Autodesk Inventor part; units mm, degrees
ref_plane "YZ Plane" through (0, 0, 0) normal (1, 0, 0) x (0, 1, 0)
ref_plane "XZ Plane" through (0, 0, 0) normal (0, 1, 0) x (-1, 0, 0)
ref_plane "XY Plane" through (0, 0, 0) normal (0, 0, 1) x (1, 0, 0)
sketch "Sketch1" plane through (0, 0, 0) normal (1, 0, 0) x (0, 1, 0)
  line L0 (348.73, -1.5913) -> (348.73, -164.0611)
  line L1 (346.8701, -168.5512) -> (220.7492, -294.6721)
  line L2 (216.2591, -296.532) -> (6.3382, -296.532)
  circle A0 centre (307.9632, 25.3963) radius 15.5575
  line L3 (348.73, -1.5913) -> (348.73, 40.2549)
  line L4 (-0.0118, -137.0094) -> (-0.0118, -290.182)
  arc A1 (-0.0118, -290.182) -> (6.3382, -296.532) centre (6.3382, -290.182) ccw
  arc A2 (216.2591, -296.532) -> (220.7492, -294.6721) centre (216.2591, -290.182) ccw
  arc A3 (346.8701, -168.5512) -> (348.73, -164.0611) centre (342.38, -164.0611) ccw
  circle A4 centre (243.0455, -117.7246) radius 14.2875
  circle A5 centre (243.0455, -117.7246) radius 38.1 construction
  circle A6 centre (140.3051, -203.2037) radius 38.1 construction
  circle A7 centre (140.3051, -203.2037) radius 14.2875
  circle A8 centre (200.1626, -272.0217) radius 2.5781
  circle A9 centre (221.1605, -257.7302) radius 14.2875
  circle A10 centre (242.1584, -243.4386) radius 2.5781
  line L5 (262.2155, 46.6049) -> (342.38, 46.6049)
  arc A11 (348.73, 40.2549) -> (342.38, 46.6049) centre (342.38, 40.2549) ccw
  line L6 (256.8542, 43.6577) -> (173.0926, -88.3121)
  line L7 (169.224, -91.0813) -> (4.8454, -130.8373)
  arc A12 (262.2155, 46.6049) -> (256.8542, 43.6577) centre (262.2155, 40.2549) ccw
  arc A13 (169.224, -91.0813) -> (173.0926, -88.3121) centre (167.7313, -84.9093) ccw
  arc A14 (4.8454, -130.8373) -> (-0.0118, -137.0094) centre (6.3382, -137.0094) ccw
  line L8 (292.4057, 46.6049) -> (191.3384, -59.565)
  point P0 (348.73, -166.6913)
  point P1 (182.4228, -257.7338)
  point P2 (269.24, 25.4)
  point P3 (171.7177, -90.4782)
  point P4 (258.7248, 46.6049)
  point P5 (-0.0118, -132.0121)
  dimension "d49" = 28.575
  dimension "d50" = 76.2
  dimension "d51" = 76.2
  dimension "d52" = 28.575
  dimension "d53" = 28.575
  dimension "d54" = 5.1562
  dimension "d56" = 6.35
  dimension "d57" = 6.35
extrude "Extrusion1" add sketch "Sketch1" along normal blind 9.525
properties part number "Intake-v2"
Build history of the part. All positions in model axes, mm. Round coordinates to 2 decimals unless told otherwise and drop trailing zeros. Loops run counter-clockwise (first coordinate to the right, second up) from the corner with the lowest first, then second, coordinate; pieces in that order, holes last. Notation, with made-up numbers: (11.5, 29) -> (36.5, 29) arc R25 ccw to (36.5, 49) -> close; hole circle Ø3 at (-30, 86.5). An arc over 180 degrees is marked (long way). Answer in a Markdown table with one row per item.
Item 1: Saw through at D-D (y = 61.5). Write the cut outline in (x, z) (3 decimals).
Answers below:
| item | result |
|---|---|
| outline | (0, -296.532) -> (9.525, -296.532) -> (9.525, -117.135) -> (0, -117.135) -> close |
Item 2: Saw through at A-A (z = -253). Write the cut outline in (x, y) (3 decimals), and give its area (3 significant figures).
Answers below:
| item | result |
|---|---|
| outline | (0, -0.012) -> (9.525, -0.012) -> (9.525, 207.679) -> (0, 207.679) -> close; (0, 234.642) -> (9.525, 234.642) -> (9.525, 262.421) -> (0, 262.421) -> close |
| area | 2,240 mm² |
Item 3: Saw through at B-B (y = 315). Write the cut outline in (x, z) (3 decimals), and give its area (3 significant figures).
Answers below:
| item | result |
|---|---|
| outline | (0, -200.421) -> (9.525, -200.421) -> (9.525, 11.521) -> (0, 11.521) -> close; (0, 39.271) -> (9.525, 39.271) -> (9.525, 46.605) -> (0, 46.605) -> close |
| area | 2,090 mm² |
Item 4: Drill centre lines: L1, parallel to Y at x = 6.75, z = -258; L2, parallel to Y at x = 6.25, z = -190; L3, parallel to Z at x = 6.75, y = 139. Where is each one in solid material? Low to high. Write a range as [from, to].
Answers below:
| item | result |
|---|---|
| L1 | y = [-0.01, 206.88], [235.45, 257.42] |
| L2 | y = [-0.01, 134.85], [145.76, 325.42] |
| L3 | z = [-296.53, -217.43], [-188.98, -98.39] |
Item 5: Pin check, flat tip, straight feed: pin 1 (17 mm diameter, centred on y = 243.05, z = -117.72, fed in from +X). Stop position of the tip, or through.
Answers below:
| item | result |
|---|---|
| pin 1 | passes through |
Item 6: Mould opens along Z. For faces 1 (the cylindrical face through (4.696, 206.887, -258.358)), 2 (the flat face through (0, 172, -161)), 3 (the flat face through (5, 302, 46.605)) say: +Z half, -Z half, draft (parallel to the pull), parting line (faces both ways), or undercut.
Answers below:
| item | result |
|---|---|
| face 1 | undercut |
| face 2 | draft |
| face 3 | +Z half |
Item 7: Saw through at C-C (x = 3.75). State how many separate pieces and enclosed holes the cut face has, and give its area (3 significant figures).
Answers below:
| item | result |
|---|---|
| separate pieces | 1 |
| enclosed holes | 6 |
| area | 75,400 mm² |
